Read the model definition and answer for the solid it produces. Units are mm, in the model's axes. A direction names the side the tool comes from. Give positions to 0.01 mm unless a question says otherwise; leave off trailing zeros. Write each loop counter-clockwise with the first axis right and the second up, starting at its lowest first coordinate (ties: lowest second). Pieces come first, ordered by that corner, then holes.
```python
from build123d import *

# Parameters (mm, degrees)
BOSS_EXTRUDE1_DEPTH     = 28.88
BOSS_EXTRUDE2_DEPTH     = 10.6
BOSS_EXTRUDE2_TAPER     = 1
BOSS_EXTRUDE3_DEPTH     = 2.35
BOSS_EXTRUDE3_TAPER     = 1
CUT_EXTRUDE1_DEPTH      = 11.2500001
CUT_EXTRUDE1_DEPTH_BACK = 11.2500001
BOSS_EXTRUDE4_DEPTH     = 1.9
BOSS_EXTRUDE4_DRAFT     = 15
SKETCH5_R               = 2.95
BOSS_EXTRUDE5_DEPTH     = 4.8
SKETCH6_OUTSIDE_W       = 73.028
SKETCH6_OUTSIDE_H       = 37.578
CUT_EXTRUDE2_DEPTH      = 4.8


with BuildPart() as part:
    # Sketch1 → Boss-Extrude1 (new body)
    with BuildSketch(Plane(origin=(0, 0, 0), x_dir=(1, 0, 0), z_dir=(0, 1, 0))):
        with BuildLine():
            Line((-18.61875, -10.25), (18.61875, -10.25))
            ThreePointArc((18.61875, -10.25), (20.302548023, -9.552548023), (21, -7.86875))
            Line((21, -7.86875), (21, 7.86875))
            ThreePointArc((21, 7.86875), (20.302548023, 9.552548023), (18.61875, 10.25))
            Line((18.61875, 10.25), (-18.61875, 10.25))
            ThreePointArc((-18.61875, 10.25), (-20.302548023, 9.552548023), (-21, 7.86875))
            Line((-21, 7.86875), (-21, -7.86875))
            ThreePointArc((-21, -7.86875), (-20.302548023, -9.552548023), (-18.61875, -10.25))
        make_face()
    extrude(amount=-BOSS_EXTRUDE1_DEPTH)

    # Sketch1_2 → Boss-Extrude2 (add)
    with BuildSketch(Plane(origin=(0, 0, 0), x_dir=(1, 0, 0), z_dir=(0, 1, 0))):
        with BuildLine():
            Line((-18.61875, -10.25), (18.61875, -10.25))
            ThreePointArc((18.61875, -10.25), (20.302548023, -9.552548023), (21, -7.86875))
            Line((21, -7.86875), (21, 7.86875))
            ThreePointArc((21, 7.86875), (20.302548023, 9.552548023), (18.61875, 10.25))
            Line((18.61875, 10.25), (-18.61875, 10.25))
            ThreePointArc((-18.61875, 10.25), (-20.302548023, 9.552548023), (-21, 7.86875))
            Line((-21, 7.86875), (-21, -7.86875))
            ThreePointArc((-21, -7.86875), (-20.302548023, -9.552548023), (-18.61875, -10.25))
        make_face()
    extrude(amount=BOSS_EXTRUDE2_DEPTH, taper=BOSS_EXTRUDE2_TAPER)

    # Sketch2 → Boss-Extrude3 (add)
    with BuildSketch(Plane(origin=(0, 0, 0), x_dir=(1, 0, 0), z_dir=(0, 1, 0))):
        with BuildLine():
            ThreePointArc((-25.778773688, 10.25), (-27.331740206, 9.606740206), (-27.975, 8.053773688))
            Line((-27.975, 8.053773688), (-27.975, 7.182744832))
            ThreePointArc((-27.975, 7.182744832), (-27.328553391, 6.247330485), (-26.225, 6.521307004))
            ThreePointArc((-26.225, 6.521307004), (-22.2, 5), (-26.225, 3.478692996))
            ThreePointArc((-26.225, 3.478692996), (-27.328553391, 3.752669515), (-27.975, 2.817255168))
            Line((-27.975, 2.817255168), (-27.975, -2.817255168))
            ThreePointArc((-27.975, -2.817255168), (-27.328553391, -3.752669515), (-26.225, -3.478692996))
            ThreePointArc((-26.225, -3.478692996), (-22.2, -5), (-26.225, -6.521307004))
            ThreePointArc((-26.225, -6.521307004), (-27.328553391, -6.247330485), (-27.975, -7.182744832))
            Line((-27.975, -7.182744832), (-27.975, -8.053773688))
            ThreePointArc((-27.975, -8.053773688), (-27.331740206, -9.606740206), (-25.778773688, -10.25))
            Line((-25.778773688, -10.25), (25.778773688, -10.25))
            ThreePointArc((25.778773688, -10.25), (27.331740206, -9.606740206), (27.975, -8.053773688))
            Line((27.975, -8.053773688), (27.975, -7.182744832))
            ThreePointArc((27.975, -7.182744832), (27.328553391, -6.247330485), (26.225, -6.521307004))
            ThreePointArc((26.225, -6.521307004), (22.2, -5), (26.225, -3.478692996))
            ThreePointArc((26.225, -3.478692996), (27.328553391, -3.752669515), (27.975, -2.817255168))
            Line((27.975, -2.817255168), (27.975, 2.817255168))
            ThreePointArc((27.975, 2.817255168), (27.328553391, 3.752669515), (26.225, 3.478692996))
            ThreePointArc((26.225, 3.478692996), (22.2, 5), (26.225, 6.521307004))
            ThreePointArc((26.225, 6.521307004), (27.328553391, 6.247330485), (27.975, 7.182744832))
            Line((27.975, 7.182744832), (27.975, 8.053773688))
            ThreePointArc((27.975, 8.053773688), (27.331740206, 9.606740206), (25.778773688, 10.25))
            Line((25.778773688, 10.25), (-25.778773688, 10.25))
        make_face()
    extrude(amount=BOSS_EXTRUDE3_DEPTH, taper=BOSS_EXTRUDE3_TAPER)

    # Sketch3 → Cut-Extrude1 (cut, two sides)
    with BuildSketch(Plane.XY) as cut_extrude1_sk:
        Polygon((20.903997143, 5.5), (13.5, 10.6), (20.814976312, 10.6), align=None)
    extrude(amount=CUT_EXTRUDE1_DEPTH, mode=Mode.SUBTRACT)
    extrude(cut_extrude1_sk.sketch, amount=-CUT_EXTRUDE1_DEPTH_BACK, mode=Mode.SUBTRACT)


with BuildPart() as boss_extrude4_tool:
    # Sketch4 → Boss-Extrude4 (with draft: the straight prism first)
    with BuildSketch(Plane(origin=(0, 10.6, 0), x_dir=(1, 0, 0), z_dir=(0, 1, 0))):
        with BuildLine():
            Line((-3.833753021, -1.5), (-2.267653421, -1.5))
            ThreePointArc((-2.267653421, -1.5), (0.185023688, -2.875), (2.637700797, -1.5))
            Line((2.637700797, -1.5), (9.685023688, -1.5))
            ThreePointArc((9.685023688, -1.5), (11.185023688, 0), (9.685023688, 1.5))
            Line((9.685023688, 1.5), (2.637700797, 1.5))
            ThreePointArc((2.637700797, 1.5), (0.185023688, 2.875), (-2.267653421, 1.5))
            Line((-2.267653421, 1.5), (-3.833753021, 1.5))
            ThreePointArc((-3.833753021, 1.5), (-17.164976312, 0), (-3.833753021, -1.5))
        make_face()
    extrude(amount=BOSS_EXTRUDE4_DEPTH)
    # Boss-Extrude4: the draft: its side faces are tilted about the plane it starts from
    boss_extrude4_sides = [boss_extrude4_tool.faces().sort_by_distance(p)[0] for p in [
        (-3.050703221, 11.55, 1.5),
        (0.185023688, 11.55, 2.875),
        (6.161362243, 11.55, 1.5),
        (11.185023688, 11.55, 0),
        (6.161362243, 11.55, -1.5),
        (0.185023688, 11.55, -2.875),
        (-3.050703221, 11.55, -1.5),
        (-17.164976312, 11.55, 0),
    ]]
    draft(boss_extrude4_sides, Plane(origin=(0, 10.6, 0), x_dir=(1, 0, 0), z_dir=(0, 1, 0)), BOSS_EXTRUDE4_DRAFT)


with BuildPart() as part_1:
    add(part.part)

    # Boss-Extrude4: add boss_extrude4_tool
    add(boss_extrude4_tool.part)

    # Sketch5 → Boss-Extrude5 (add)
    with BuildSketch(Plane(origin=(0, 12.5, 0), x_dir=(1, 0, 0), z_dir=(0, 1, 0))):
        with Locations((-10.414976312, 0)):
            Circle(SKETCH5_R)
    extrude(amount=BOSS_EXTRUDE5_DEPTH)

    # Sketch6 outside → Cut-Extrude2 (cut)
    with BuildSketch(Plane(origin=(0, 12.5, 0), x_dir=(1, 0, 0), z_dir=(0, 1, 0))):
        Rectangle(SKETCH6_OUTSIDE_W, SKETCH6_OUTSIDE_H)
        Polygon((-9.183129599, -2.240720851), (-8.681009817, -2.386600133), (-8.664585713, -1.863976666), (-8.141962246, -1.88040077), (-8.256025306, -1.370111971), (-7.745736507, -1.25604891), (-7.983119731, -0.790158102), (-7.517228922, -0.552774878), (-7.863016648, -0.160555693), (-7.470797463, 0.185232033), (-7.903262576, 0.47913502), (-7.609359589, 0.911600133), (-8.101328716, 1.088719918), (-7.924208932, 1.580689045), (-8.444769843, 1.629896539), (-8.395562349, 2.150457451), (-8.912006289, 2.068660767), (-8.993802973, 2.585104706), (-9.473679868, 2.37744343), (-9.681341145, 2.857320325), (-10.094498566, 2.536842579), (-10.414976312, 2.95), (-10.735454058, 2.536842579), (-11.148611479, 2.857320325), (-11.356272755, 2.37744343), (-11.83614965, 2.585104706), (-11.917946335, 2.068660767), (-12.434390274, 2.150457451), (-12.38518278, 1.629896539), (-12.905743692, 1.580689045), (-12.728623908, 1.088719918), (-13.220593035, 0.911600133), (-12.926690047, 0.47913502), (-13.359155161, 0.185232033), (-12.966935976, -0.160555693), (-13.312723701, -0.552774878), (-12.846832893, -0.790158102), (-13.084216117, -1.25604891), (-12.573927317, -1.370111971), (-12.687990378, -1.88040077), (-12.16536691, -1.863976666), (-12.148942806, -2.386600133), (-11.646823024, -2.240720851), (-11.500943742, -2.742840633), (-11.050877679, -2.476672305), (-10.784709351, -2.926738369), (-10.414976312, -2.55700533), (-10.045243273, -2.926738369), (-9.779074945, -2.476672305), (-9.329008881, -2.742840633), align=None, mode=Mode.SUBTRACT)
    extrude(amount=CUT_EXTRUDE2_DEPTH, mode=Mode.SUBTRACT)


solid = part_1.part
```
Item 1: Section C-C (x = 18) is taken. Write down the section's boundary in (y, z), and give its area (3 significant figures).
Result set:
outline: (-28.88, -10.25) - (0, -10.25) - (7.5, -10.12) - (7.5, 10.12) - (0, 10.25) - (-28.88, 10.25) - close
area: 745 mm2
Item 2: Section A-A (y = -15.5) is taken. Write down the section's boundary in (x, z), and give its area (3 significant figures).
Result set:
outline: (-21, -7.87) arc R2.38 ccw to (-18.62, -10.25) - (18.62, -10.25) arc R2.38 ccw to (21, -7.87) - (21, 7.87) arc R2.38 ccw to (18.62, 10.25) - (-18.62, 10.25) arc R2.38 ccw to (-21, 7.87) - close
area: 856 mm2
Item 3: Find the intervals of material crossed by line 1 along Z through (x, y) = (-24.5, 1); line 2 along X through (y, z) = (14.5, -2.75); line 3 along X through (y, z) = (-26, -5.5), in increasing order.
Result set:
line 1: z = -10.23 to -7.32, -2.68 to 2.68, 7.32 to 10.23
line 2: x = -11.2 to -11.01, -10.57 to -10.26, -9.82 to -9.63
line 3: x = -21 to 21
Item 4: Section B-B (x = 24.5) is taken. Give the number of separate pieces and of enclosed holes in the cut face, and give its area (3 significant figures).
Result set:
separate pieces: 3
enclosed holes: 0
area: 26.3 mm2
Item 5: Which of the six approach directions +Z, -Z, +X, -X, +Y, -Y give full straight-line access (tool end or side, diameter ignored) to faces 4 (the cylindrical face through (-20.284, -14.238, -9.571)), 5 (the cylindrical face through (20.321, -14.238, -9.534)), 6 (the conical face through (-20.239, 6.533, 9.454)), 7 (the flat face through (6.06, 11.54, -1.25)), 8 (the cylindrical face through (-20.321, -14.238, 9.534))?
Result set:
face 4: -Z, -X, -Y
face 5: -Z, +X, -Y
face 6: +Z, -X, +Y
face 7: -Z, +X, +Y
face 8: +Z, -X, -Y
Item 6: Each of these flat-tipped pins is pushed along its axis until it touches: pin 1 Ø10 at (x, z) = (23, -2) entering from +Y; pin 2 Ø2 at (x, z) = (-9, -4) entering from +Y; pin 3 Ø8 at (y, z) = (5, 6.5) entering from -X. Where does it stop, or does it pass through?
Result set:
pin 1: stops at y = 7.5
pin 2: stops at y = 12.5
pin 3: stops at x = -27.96
Item 7: Determine the mould class of faces 1 (the cylindrical face through (20.284, -14.238, 9.571)), 2 (the conical face through (-27.33, 1.19, 9.58)), 3 (the conical face through (-22.18, 1.19, 4.92)) for opening direction X: pulls with the +X half, pulls with the -X half, needs draft (parallel to the pull), parting line crosses it, or undercut.
Result set:
face 1: pulls with the +X half
face 2: pulls with the -X half
face 3: undercut
